Autodesk Fusion 360 part; units mm, degrees
sketch "Sketch1" plane through (0, 0, 0) normal (0, 1, 0) x (1, 0, 0)
  circle A0 centre (0, 0) radius 35
  circle A1 centre (0, 0) radius 14
  dimension "d1" = 70
  dimension "d2" = 28
extrude "Extrude1" add sketch "Sketch1" along normal blind 10
sketch "Sketch2" plane through (0, 10, 0) normal (0, 1, 0) x (-1, 0, 0)
  circle A0 centre (0, 0) radius 14
  circle A1 centre (0, 0) radius 35
  circle A2 centre (0, 0) radius 16.5
  circle A3 centre (0, 0) radius 21
  circle A4 centre (0, 0) radius 25 construction
  circle A5 centre (0, -25) radius 4
  line L0 (0, 0) -> (0, -25) construction
  line L1 (0, 1.75) -> (0, 22.5)
  circle A6 centre (25, 0) radius 4
  circle A7 centre (0, 25) radius 4
  circle A8 centre (-25, 0) radius 4
  dimension "d5" = 33
  dimension "d6" = 42
  dimension "d7" = 50
  dimension "d8" = 8
  dimension "d10" = 360
extrude "Extrude2" add sketch "Sketch2" along normal blind 5 contours A3
extrude "Extrude3" cut sketch "Sketch2" against normal blind 10 contours A7 | A6 | A5 | A8
For this review, take the finished solid that the model builds, in its own axes (mm). A direction names the side the tool comes from. Coordinates: 2 decimals unless noted, no trailing zeros. Loops run counter-clockwise (first coordinate to the right, second up) from the corner with the lowest first, then second, coordinate; pieces in that order, holes last. Notation, with made-up numbers: (7.5, 28) - (12.5, 28) arc R35 cw to (12.5, 62) - close; hole circle Ø4 at (12.5, -15.5). An arc over 180 degrees is marked (long way). Use one line per item in the form item = value. Start each with the question number.
1) Take a section at D-D (x = -20). State the section outline as (y, z) points, plus the area to 3 significant figures.
2) Take a section at C-C (y = 4). State the section outline as (x, z) points.
3) To check wall thickness, follow probe 1 along Z at (x, y) = (0, 6.25); probe 2 along Z at (x, y) = (0, 12.55). State the ranges of each line that lie inside material, in increasing order. Write a range as from..to.
4) Take a section at A-A (x = -27.5). State the section outline as (y, z) points.
5) Take a section at B-B (z = -25). State the section outline as (x, y) points.
6) Draft analysis for pull direction Z (two halves, no side actions). For faces 1 (the face through (0.521, 5.07, 28.966)), 2 (the face through (-20.03, 12.46, -6.31)), 3 (the face through (13, 15, -11)), state which applies: released by +Z, released by -Z, zero draft, split by the parting line, or undercut.
7) For pin 1 (4 mm diameter, centred on y = 10.5, z = -17.5, fed in from +X); pin 2 (1 mm diameter, centred on y = 10, z = -16.5, fed in from +X); pin 3 (5 mm diameter, centred on x = -12.5, y = 2.5, fed in from -Z), all flat-tipped, find the tip position at first contact; note any pin that passes through.
8) For faces 4 (the face through (12.932, 4.93, -5.362)), 5 (the face through (15, 10, 15)), list the 3-axis set-ups (+Z, -Z, +X, -X, +Y, -Y) from which the entire face can be reached by the end or side of a thin tool; tool diameter is ignored.
From the geometry:
q1.outline = (0, -28.72) - (10, -28.72) - (10, -6.4) - (15, -6.4) - (15, 6.4) - (10, 6.4) - (10, 28.72) - (0, 28.72) - close
q1.area = 638 mm2
q2.outline = circle Ø70 at (0, 0); hole circle Ø8 at (-25, 0); hole circle Ø28 at (0, 0); hole circle Ø8 at (0, -25); hole circle Ø8 at (0, 25); hole circle Ø8 at (25, 0)
q3.probe_1 = -35..-29, -21..-14, 14..21, 29..35
q3.probe_2 = -21..-16.5, 16.5..21
q4.outline = (0, -21.65) - (10, -21.65) - (10, -3.12) - (0, -3.12) - close; (0, 3.12) - (10, 3.12) - (10, 21.65) - (0, 21.65) - close
q5.outline = (-24.49, 0) - (-4, 0) - (-4, 10) - (-24.49, 10) - close; (4, 0) - (24.49, 0) - (24.49, 10) - (4, 10) - close
q6.face_1 = undercut
q6.face_2 = split by the parting line
q6.face_3 = zero draft
q7.pin_1 = 31.35
q7.pin_2 = 31.13
q7.pin_3 = -33.54
q8.face_4 = +Y, -Y
q8.face_5 = +Y
